Print and shaded views of the part. All mm, measured from the part's lowest x, y and z. A direction names the side the tool comes from. Give positions to 0.01 mm unless a question says otherwise; leave off trailing zeros. Order: outer loops, then holes, each group sorted by start corner. A loop starts at its lowest first (then second) coordinate and runs counter-clockwise, first axis right, second up. Notation, with made-up numbers: (-26, -33) -> (7, -33) arc R17 cw to (7, -19) -> close; hole circle Ø6 at (76, 82). An arc over 180 degrees is marked (long way). One line per question, with ' | ' between items. Start each with the question number.
(1) Drill centre lines: L1, parallel to Z at x = 7.25, y = 5.5; L2, parallel to X at y = 5.25, z = 4; L3, parallel to X at y = 0.75, z = 3.25. Where is each one in solid material? Low to high. Write a range as from..to.
(2) Cut at C-C (y = 7.5). Give the cut face in (x, z), then the cut area to 3 significant figures.
(3) Cut at A-A (x = 3.8). Give the cut face in (y, z).
(4) Pull direction Z, two halves, no side cores. Call the marked faces 1, 2 and 3: +Z half, -Z half, draft (parallel to the pull), parting line (faces both ways), or undercut.
(5) Pin check, flat tips, straight feed: pin 1 Ø2 at (y, z) = (6, 5) entering from -X; pin 2 Ø2 at (y, z) = (5.5, 5) entering from +X; pin 3 Ø3 at (y, z) = (1.5, 5.5) entering from -X. Stop position of each tip, or through.
(6) Cut at D-D (y = 1.25). Give the cut face in (x, z).
(7) Which spindle directions (+Z, -Z, +X, -X, +Y, -Y) get a long thin tool onto all of the face, cutting with end or side? Do the marked faces 4, 5 and 6. Say none if no direction does.
(8) Cut at B-B (z = 3.3). Give the cut face in (x, y).
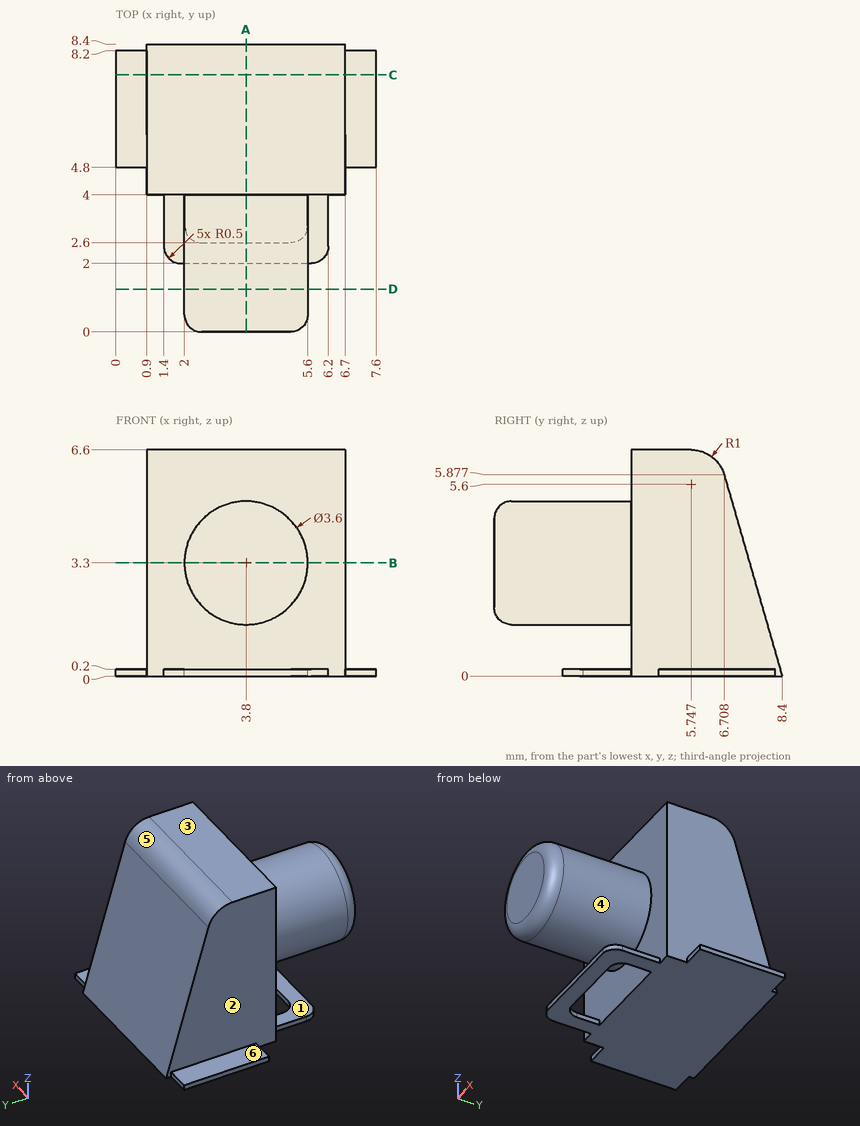
Result set:
1) L1: z = 0..0.2 | L2: x = 0.9..6.7 | L3: x = 2..5.6
2) outline: (0, 0) -> (7.6, 0) -> (7.6, 0.2) -> (6.7, 0.2) -> (6.7, 3.13) -> (0.9, 3.13) -> (0.9, 0.2) -> (0, 0.2) -> close | area: 18.5 mm2
3) outline: (0, 2) arc R0.5 ccw to (0.5, 1.5) -> (4, 1.5) -> (4, 0) -> (8.4, 0) -> (6.71, 5.88) arc R1 ccw to (5.75, 6.6) -> (4, 6.6) -> (4, 5.1) -> (0.5, 5.1) arc R0.5 ccw to (0, 4.6) -> close; (2, 0) -> (2.6, 0) -> (2.6, 0.2) -> (2, 0.2) -> close
4) face 1: undercut | face 2: draft | face 3: +Z half
5) pin 1: stops at x = 0.9 | pin 2: stops at x = 6.7 | pin 3: stops at x = 2.14
6) outline: circle Ø3.6 at (3.8, 3.3)
7) face 4: -Y | face 5: +Z, +X, -X, +Y | face 6: +Z, -X, +Y, -Y
8) outline: (0.9, 4) -> (2, 4) -> (2, 0.5) arc R0.5 ccw to (2.5, 0) -> (5.1, 0) arc R0.5 ccw to (5.6, 0.5) -> (5.6, 4) -> (6.7, 4) -> (6.7, 7.45) -> (0.9, 7.45) -> close
